```python
from build123d import *

# Parameters (mm, degrees)
CHAMFER1_SIZE           = 0.25
BOSS_EXTRUDE1_START     = -2
SKETCH2_R               = 44.5
BOSS_EXTRUDE1_DEPTH     = 2
CUT_EXTRUDE3_DEPTH      = 93.051684706
CUT_EXTRUDE3_DEPTH_BACK = 93.051684706
SKETCH4_W               = 115.72626858
SKETCH4_H               = 18.336467462
CHAMFER2_SIZE           = 0.25


with BuildPart() as part:
    # Sketch1 → Revolve1 (revolve)
    with BuildSketch(Plane(origin=(0, 0, 0), x_dir=(1, 0, 0), z_dir=(0, 1, 0)), mode=Mode.PRIVATE) as revolve1_sk:
        Polygon((37.85, 0), (37.85, -18.7), (44.5, -18.7), (44.5, -16.2), (43.5, -16.2), (43.5, -11.2), (44.5, -11.2), (44.5, -8.7), (55.25, -8.7), (55.25, -6.7), (39.85, -6.7), (39.85, 0), align=None)
    revolve(revolve1_sk.sketch.rotate(Axis((0, 0, -73.981367368), (0, 0, 1)), 180), axis=Axis((0, 0, -73.981367368), (0, 0, 1)))

    # Chamfer1
    chamfer1_edges = [part.edges().sort_by_distance(p)[0] for p in [
        (44.5, 0, 11.2),
        (43.5, 0, 11.2),
        (43.5, 0, 16.2),
        (44.5, 0, 16.2),
    ]]
    chamfer(chamfer1_edges, length=CHAMFER1_SIZE)

    # Sketch2 → Boss-Extrude1 (add)
    with BuildSketch(Plane.XY.offset(8.7).offset(BOSS_EXTRUDE1_START)):
        with BuildLine():
            Line((9.797958971, 59.25), (33.217958971, 59.25))
            Line((33.217958971, 59.25), (67.92098466, -0.857403669))
            Line((67.92098466, -0.857403669), (56.21098466, -21.139718626))
            ThreePointArc((56.21098466, -21.139718626), (47.847903559, -27.625), (46.413025689, -38.110281374))
            Line((46.413025689, -38.110281374), (34.703025689, -58.392596331))
            Line((34.703025689, -58.392596331), (-34.703025689, -58.392596331))
            Line((-34.703025689, -58.392596331), (-46.413025689, -38.110281374))
            ThreePointArc((-46.413025689, -38.110281374), (-47.847903559, -27.625), (-56.21098466, -21.139718626))
            Line((-56.21098466, -21.139718626), (-67.92098466, -0.857403669))
            Line((-67.92098466, -0.857403669), (-33.217958971, 59.25))
            Line((-33.217958971, 59.25), (-9.797958971, 59.25))
            ThreePointArc((-9.797958971, 59.25), (0, 55.25), (9.797958971, 59.25))
        make_face()
        with Locations(Location((0, 0, 0), (0, 0, 180))):
            Circle(SKETCH2_R, mode=Mode.SUBTRACT)
    extrude(amount=BOSS_EXTRUDE1_DEPTH)

    # Sketch4 → Cut-Extrude3 (cut, two sides: drawn at the far end of the back side and taken through both)
    with BuildSketch(Plane(origin=(0, 0, 0), x_dir=(1, 0, 0), z_dir=(0, 1, 0)).offset(-CUT_EXTRUDE3_DEPTH_BACK)):
        with Locations((0.509486717, -17.868233731)):
            Rectangle(SKETCH4_W, SKETCH4_H)
    extrude(amount=CUT_EXTRUDE3_DEPTH + CUT_EXTRUDE3_DEPTH_BACK, mode=Mode.SUBTRACT)

    # Chamfer2
    chamfer2_edges = [part.edges().sort_by_distance(p)[0] for p in [
        (39.85, 0, 0),
    ]]
    chamfer(chamfer2_edges, length=CHAMFER2_SIZE)


solid = part.part
```
Check sheet for the modelled part. Datum: model origin and axes. Units: mm. A direction names the side the tool comes from. Round coordinates to 2 decimals unless told otherwise and drop trailing zeros. Order: outer loops, then holes, each group sorted by start corner. A loop starts at its lowest first (then second) coordinate and runs counter-clockwise, first axis right, second up. Notation, with made-up numbers: M -21.75,-20 L 1.25,-20 A22 cw 1.25,-2 Z; hole C -33,54 d6. An arc over 180 degrees is marked long. Answer in a Markdown table with one row per item.
(1) Set-up check for faces 1 (the flat face through (31, 27, 6.7)), 2 (the flat face through (-50.8, 28.8, 7.7)): record each of +Z, -Z, +X, -X, +Y, -Y from which the full face is reachable in a straight line by a thin tool's end or side.
Findings:
| item | result |
|---|---|
| face 1 | -Z |
| face 2 | +Z, -Z, -X, +Y |
(2) Section check D-D on x = -48. Record the boundary of the cut face in (y, z), plus the area to 3 significant figures.
Findings:
| item | result |
|---|---|
| outline | M -27.37,6.7 L 33.65,6.7 L 33.65,8.7 L -27.37,8.7 Z |
| area | 122 mm^2 |
(3) Draft check along Y on faces 3 (the cylindrical face through (-47.77, -27.76, 7.69)), 4 (the flat face through (1, -38, 8.7)), 5 (the cylindrical face through (-38, -12, 3)). Enter one of: +Y half, -Y half, draft (parallel to the pull), parting line (faces both ways), or undercut.
Findings:
| item | result |
|---|---|
| face 3 | undercut |
| face 4 | draft |
| face 5 | parting line |
(4) Section check C-C on y = -47.5. Record the boundary of the cut face in (x, z), plus the area to 3 significant figures.
Findings:
| item | result |
|---|---|
| outline | M -40.99,6.7 L 40.99,6.7 L 40.99,8.7 L -40.99,8.7 Z |
| area | 164 mm^2 |
(5) Section check B-B on z = 3. Record the boundary of the cut face in (x, y).
Findings:
| item | result |
|---|---|
| outline | C 0,0 d79.7; hole C 0,0 d75.7 |
(6) Section check A-A on x = 0. Record the boundary of the cut face in (y, z), plus the area to 3 significant figures.
Findings:
| item | result |
|---|---|
| outline | M -58.39,6.7 L -39.85,6.7 L -39.85,0.25 L -39.6,0 L -37.85,0 L -37.85,8.7 L -58.39,8.7 Z; M 37.85,0 L 39.6,0 L 39.85,0.25 L 39.85,6.7 L 55.25,6.7 L 55.25,8.7 L 37.85,8.7 Z |
| area | 103 mm^2 |
(7) Material ranges on line 1 along Y through (x, z) = (0, 2.75); line 2 along Y through (x, z) = (0, 7); line 3 along Z through (x, y) = (-2.5, 41), recorded low to high. Write a range as from..to.
Findings:
| item | result |
|---|---|
| line 1 | y = -39.85..-37.85, 37.85..39.85 |
| line 2 | y = -58.39..-37.85, 37.85..55.25 |
| line 3 | z = 6.7..8.7 |
(8) Gauge pin test, flat ends, axial feed: pin 1 (5 mm diameter, centred on x = -6, y = -36, fed in from +Z); pin 2 (3 mm diameter, centred on y = -22.5, z = 4.5, fed in from -X); pin 3 (3 mm diameter, centred on x = 7, z = 5, fed in from +Y); pin 4 (3 mm diameter, centred on y = -15.5, z = 4, fed in from +X). Record the tip position at first contact, or that the pin passes through.
Findings:
| item | result |
|---|---|
| pin 1 | stops at z = 8.7 |
| pin 2 | stops at x = -33.87 |
| pin 3 | stops at y = 39.47 |
| pin 4 | stops at x = 37.31 |
